Autodesk Inventor part; units mm, degrees
ref_plane "YZ Plane" through (0, 0, 0) normal (1, 0, 0) x (0, 1, 0)
ref_plane "XZ Plane" through (0, 0, 0) normal (0, 1, 0) x (-1, 0, 0)
ref_plane "XY Plane" through (0, 0, 0) normal (0, 0, 1) x (1, 0, 0)
sketch "Sketch1" plane through (0, 0, 0) normal (0, 1, 0) x (-1, 0, 0)
  line L0 (12.2137, 18.6426) -> (-13.1863, 18.6426)
  line L1 (-13.1863, 18.6426) -> (-13.1863, -19.4574)
  line L2 (-13.1863, -19.4574) -> (12.2137, -19.4574)
  line L3 (12.2137, -19.4574) -> (12.2137, 18.6426)
  point P0 (0, 0)
  dimension "d0" = 25.4
  dimension "d1" = 38.1
extrude "Extrusion1" add sketch "Sketch1" along normal blind 0.635
hole "Hole1" at (9.5986, 0.635, 13.8801) direction (0, -1, 0) diameter 4.4958 depth 0.635
hole "Hole2" at (-8.6259, 0.635, 13.8801) direction (0, -1, 0) diameter 4.4958 depth 0.635
hole "Hole3" at (-8.6259, 0.635, -14.6949) direction (0, -1, 0) diameter 4.4958 depth 0.635
hole "Hole4" at (9.5986, 0.635, -14.6949) direction (0, -1, 0) diameter 4.4958 depth 0.635
properties part number "Shielding"
Part model, mm, in its own coordinate system. Coordinates: 2 decimals unless noted, no trailing zeros. Write each loop counter-clockwise with the first axis right and the second up, starting at its lowest first coordinate (ties: lowest second). Pieces come first, ordered by that corner, then holes.
Item 1: Pin check, flat tip, straight feed: pin 1 (4 mm diameter, centred on x = 9.6, z = 13.88, fed in from -Y). Stop position of the tip, or through.
Item 2: Mould opens along Z. For faces 1 (the face through (1, 0.635, 0)), 2 (the face through (-10.145, 0.313, 12.223)) say: released by +Z, released by -Z, zero draft, split by the parting line, or undercut.
Item 3: Slice it at B-B (z = 13). Write the cut outline in (x, y) (3 decimals).
Item 4: Slice it at C-C (y = 0.25). Write the cut outline in (x, z), and give its area (3 significant figures).
Item 5: Probe line 1 (Z direction, x = -8.5, y = 0.25); line 2 (X direction, y = 0.55, z = 14); line 3 (X direction, y = 0.1, z = -16). List the from-to ranges inside material, lowest first.
Item 6: Slice it at A-A (x = 7.75). Write the cut outline in (y, z) (3 decimals), and give its area (3 significant figures).
Results found:
1. pin 1: passes through
2. face 1: zero draft
2. face 2: undercut
3. outline: (-12.214, 0) - (-10.694, 0) - (-10.694, 0.635) - (-12.214, 0.635) - close; (-6.557, 0) - (7.53, 0) - (7.53, 0.635) - (-6.557, 0.635) - close; (11.667, 0) - (13.186, 0) - (13.186, 0.635) - (11.667, 0.635) - close
4. outline: (-12.21, -19.46) - (13.19, -19.46) - (13.19, 18.64) - (-12.21, 18.64) - close; hole circle Ø4.5 at (-8.63, -14.69); hole circle Ø4.5 at (-8.63, 13.88); hole circle Ø4.5 at (9.6, -14.69); hole circle Ø4.5 at (9.6, 13.88)
4. area: 904 mm2
5. line 1: z = -19.46 to -16.94, -12.45 to 11.64, 16.12 to 18.64
5. line 2: x = -12.21 to -10.87, -6.38 to 7.35, 11.84 to 13.19
5. line 3: x = -12.21 to -10.46, -6.8 to 7.77, 11.43 to 13.19
6. outline: (0, -19.457) - (0.635, -19.457) - (0.635, -15.974) - (0, -15.974) - close; (0, -13.416) - (0.635, -13.416) - (0.635, 12.601) - (0, 12.601) - close; (0, 15.159) - (0.635, 15.159) - (0.635, 18.643) - (0, 18.643) - close
6. area: 20.9 mm2
